Here's the drawing with two shaded views (mm, measured from the low corner). I have some questions. A direction names the side the tool comes from. Coordinates: 2 decimals unless noted, no trailing zeros. Write each loop counter-clockwise with the first axis right and the second up, starting at its lowest first coordinate (ties: lowest second). Pieces come first, ordered by that corner, then holes.
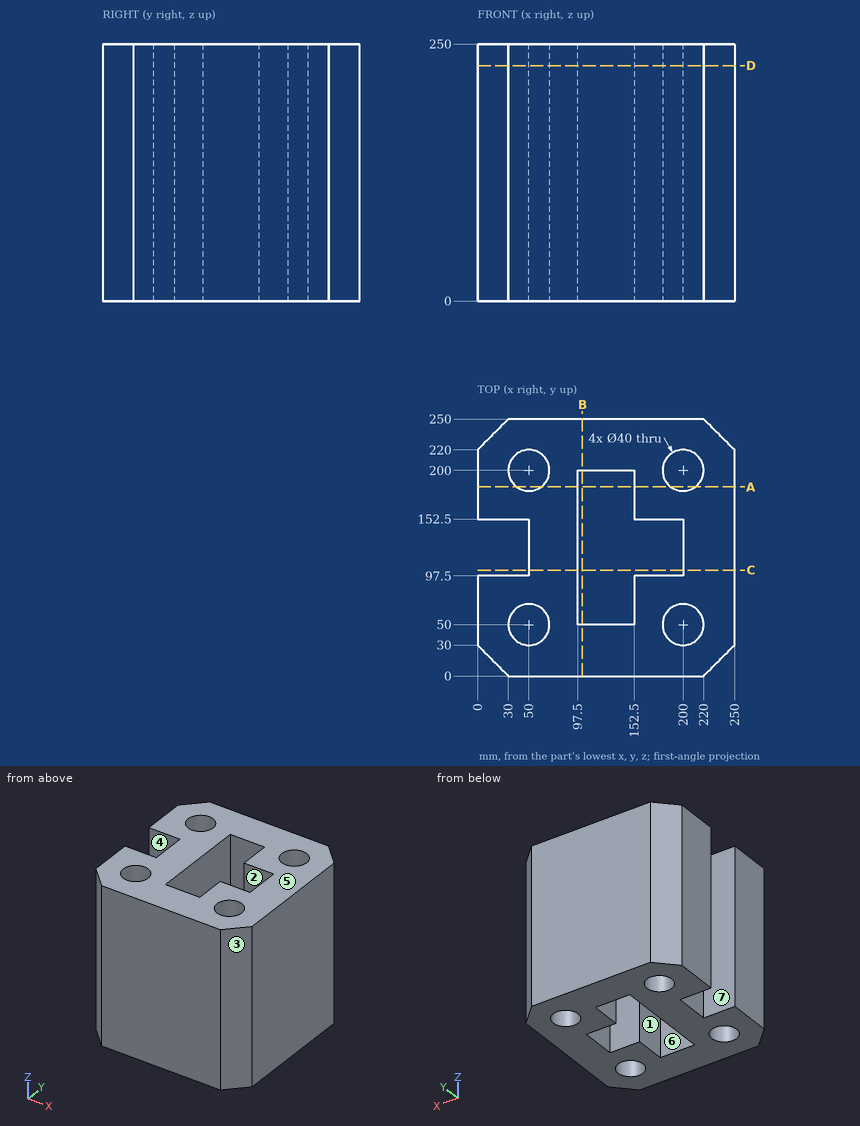
1. I want a section at B-B on x = 102. Please give me the cut outline in (y, z), plus the area to 3 significant figures.
Verdict:
outline: (0, 0) - (50, 0) - (50, 250) - (0, 250) - close; (200, 0) - (250, 0) - (250, 250) - (200, 250) - close
area: 25,000 mm2
2. Please list where these lines run through material, in increasing order: line 1 along X through (y, z) = (121.5, 170); line 2 along Y through (x, z) = (178, 104.5); line 3 along Y through (x, z) = (102.5, 168.5).
Verdict:
line 1: x = 50 to 97.5, 200 to 250
line 2: y = 0 to 97.5, 152.5 to 250
line 3: y = 0 to 50, 200 to 250
3. I want a section at D-D on z = 229. Please give me the cut outline in (x, y).
Verdict:
outline: (0, 30) - (30, 0) - (220, 0) - (250, 30) - (250, 220) - (220, 250) - (30, 250) - (0, 220) - (0, 152.5) - (50, 152.5) - (50, 97.5) - (0, 97.5) - close; hole circle Ø40 at (50, 50); hole circle Ø40 at (50, 200); hole (97.5, 50) - (152.5, 50) - (152.5, 97.5) - (200, 97.5) - (200, 152.5) - (152.5, 152.5) - (152.5, 200) - (97.5, 200) - close; hole circle Ø40 at (200, 50); hole circle Ø40 at (200, 200)
4. I want a section at A-A on y = 184. Please give me the cut outline in (x, z), plus the area to 4 significant figures.
Verdict:
outline: (0, 0) - (38, 0) - (38, 250) - (0, 250) - close; (62, 0) - (97.5, 0) - (97.5, 250) - (62, 250) - close; (152.5, 0) - (188, 0) - (188, 250) - (152.5, 250) - close; (212, 0) - (250, 0) - (250, 250) - (212, 250) - close
area: 36,750 mm2
5. I want a section at C-C on y = 103. Please give me the cut outline in (x, z), plus the area to 3 significant figures.
Verdict:
outline: (50, 0) - (97.5, 0) - (97.5, 250) - (50, 250) - close; (200, 0) - (250, 0) - (250, 250) - (200, 250) - close
area: 24,400 mm2
6. If we mould it in two halves opening along X, with no side actions, what happens to the marked faces 1, 2, 3 and 4? For each: pulls with the +X half, pulls with the -X half, needs draft (parallel to the pull), parting line crosses it, or undercut.
Verdict:
face 1: undercut
face 2: undercut
face 3: pulls with the +X half
face 4: needs draft
7. On a 3-axis mill with a long thin cutter (end or side, diameter ignored), from which of +Z, -Z, +X, -X, +Y, -Y can I reach the whole of each face in a straight line? I mean the marked faces 5, 6 and 7. Say none if no direction works.
Verdict:
face 5: +Z, +X, -X, +Y, -Y
face 6: +Z, -Z
face 7: +Z, -Z, -X
